Geometry: final body of the model. Coordinates: model frame, mm. Face numbers are marked on the shaded views. A direction names the side the tool comes from. Give positions to 0.01 mm unless a question says otherwise; leave off trailing zeros. Write each loop counter-clockwise with the first axis right and the second up, starting at its lowest first coordinate (ties: lowest second). Pieces come first, ordered by that corner, then holes. Notation, with made-up numbers: (-15.75, -34) -> (42.25, -34) arc R10 ccw to (42.25, -29) -> close; hole circle Ø9 at (-33.75, 52.5). An arc over 180 degrees is marked (long way). Answer in a Markdown table with one row per item. Add a question column.
Item 1: Section query D-D on x = -127.5. Output: boundary loops of the cut face in (y, z).
Item 2: Section query A-A on z = -30. Output: boundary loops of the cut face in (x, y).
Item 3: First-contact query: P1, Ø4.5, axis at x = -64.5, y = -155, coming from the +Z side. Flat tip, straight axial feed; report the tip coordinate or a pass-through.
Item 4: Draft query along Y for the marked faces 3, 4 and 5. Return one class per face: +Y half, -Y half, draft (parallel to the pull), parting line (faces both ways), or undercut.
Item 5: Material intervals for probe 1 along X at (y, z) = (-83, -213); probe 2 along Y at (x, z) = (-166.5, -226); probe 3 along Z at (x, y) = (99.5, 5), sorted ascending. Write a range as from..to.
Item 6: Section query C-C on z = -123.5. Output: boundary loops of the cut face in (x, y), plus the area to 3 significant figures.
Item 7: Access query for the marked faces 1 and 2. Directions: +Z, -Z, +X, -X, +Y, -Y. A direction counts if a zero-diameter tool reaches every point of the face in a straight line with its end or side. Return the directions, or none.
Item 8: Section query B-B on y = -12.5. Output: boundary loops of the cut face in (x, z), plus the area to 3 significant figures.
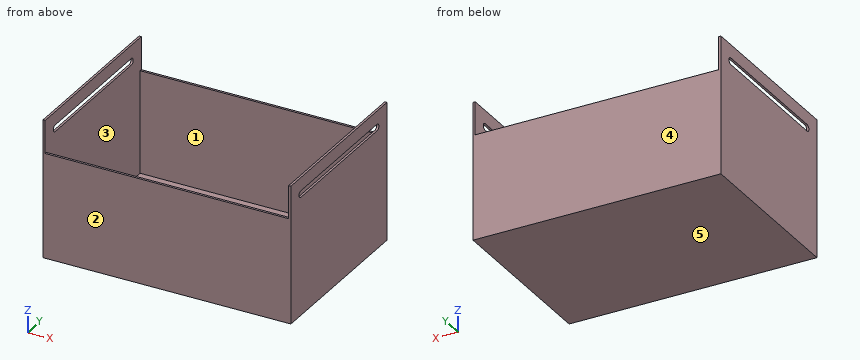
```python
from build123d import *

# Parameters (mm, degrees)
SKETCH_1_W          = 450
SKETCH_1_H          = 315
EXTRUDE_1_DEPTH     = 250
SHELL_3_T           = -4
SKETCH_4_W          = 442
SKETCH_4_H          = 60
CUT_EXTRUDE_1_DEPTH = 316
CUT_EXTRUDE_2_DEPTH = 451


with BuildPart() as part:
    # 草图1 → 凸台-拉伸1 (new body)
    with BuildSketch(Plane.XY):
        Rectangle(SKETCH_1_W, SKETCH_1_H)
    extrude(amount=-EXTRUDE_1_DEPTH)

    # 抽壳3
    shell_3_openings = [part.faces().sort_by_distance(p)[0] for p in [
        (0, 0, 0),
    ]]
    offset(amount=SHELL_3_T, openings=shell_3_openings, kind=Kind.INTERSECTION)

    # 草图4 → 切除-拉伸1 (cut, through all)
    with BuildSketch(Plane.XZ.offset(157.5)):
        with Locations((0, -30)):
            Rectangle(SKETCH_4_W, SKETCH_4_H)
    extrude(amount=-CUT_EXTRUDE_1_DEPTH, mode=Mode.SUBTRACT)

    # 草图5 → 切除-拉伸2 (cut, through all)
    with BuildSketch(Plane(origin=(225, 0, 0), x_dir=(0, 0, -1), z_dir=(1, 0, 0))):
        with BuildLine():
            Line((36, 125), (36, -125))
            ThreePointArc((36, -125), (30, -131), (24, -125))
            Line((24, -125), (24, 125))
            ThreePointArc((24, 125), (30, 131), (36, 125))
        make_face()
    extrude(amount=-CUT_EXTRUDE_2_DEPTH, mode=Mode.SUBTRACT)


solid = part.part
```
Findings below:
| question | item | result |
|---|---|---|
| 1 | outline | (-157.5, -250) -> (157.5, -250) -> (157.5, -60) -> (153.5, -60) -> (153.5, -246) -> (-153.5, -246) -> (-153.5, -60) -> (-157.5, -60) -> close |
| 2 | outline | (-225, -157.5) -> (-221, -157.5) -> (-221, -131) -> (-225, -131) -> close; (-225, 131) -> (-221, 131) -> (-221, 157.5) -> (-225, 157.5) -> close; (221, -157.5) -> (225, -157.5) -> (225, -131) -> (221, -131) -> close; (221, 131) -> (225, 131) -> (225, 157.5) -> (221, 157.5) -> close |
| 3 | P1 | stops at z = -60 |
| 4 | face 3 | undercut |
| 4 | face 4 | +Y half |
| 4 | face 5 | draft |
| 5 | probe 1 | x = -225..-221, 221..225 |
| 5 | probe 2 | y = -157.5..-153.5, 153.5..157.5 |
| 5 | probe 3 | z = -250..-246 |
| 6 | outline | (-225, -157.5) -> (225, -157.5) -> (225, 157.5) -> (-225, 157.5) -> close; hole (-221, -153.5) -> (221, -153.5) -> (221, 153.5) -> (-221, 153.5) -> close |
| 6 | area | 6,060 mm^2 |
| 7 | face 1 | +Z |
| 7 | face 2 | +Z, -Z, +X, -X, -Y |
| 8 | outline | (-225, -250) -> (225, -250) -> (225, -36) -> (221, -36) -> (221, -246) -> (-221, -246) -> (-221, -36) -> (-225, -36) -> close; (-225, -24) -> (-221, -24) -> (-221, 0) -> (-225, 0) -> close; (221, -24) -> (225, -24) -> (225, 0) -> (221, 0) -> close |
| 8 | area | 3,670 mm^2 |
